Geometry check sheet. Reference: the model listing, model coordinates, mm. A direction names the side the tool comes from. Give positions to 0.01 mm unless a question says otherwise; leave off trailing zeros. Loops run counter-clockwise (first coordinate to the right, second up) from the corner with the lowest first, then second, coordinate; pieces in that order, holes last. Notation, with made-up numbers: (8.5, 37) -> (61.5, 37) arc R30 cw to (61.5, 61) -> close; hole circle Ø7 at (-6, 84.25). An arc over 180 degrees is marked (long way). Answer in a Markdown table with one row per item. Add a question column.
```python
from build123d import *

# Parameters (mm, degrees)
SKETCH1_R           = 5
BOSS_EXTRUDE1_DEPTH = 10
SKETCH2_R           = 8.5
BOSS_EXTRUDE2_DEPTH = 5
CUT_EXTRUDE1_DEPTH  = 3
CHAMFER1_SIZE       = 4


with BuildPart() as part:
    # Sketch1 → Boss-Extrude1 (new body)
    with BuildSketch(Plane.XY):
        Circle(SKETCH1_R)
    extrude(amount=BOSS_EXTRUDE1_DEPTH)

    # Sketch2 → Boss-Extrude2 (add)
    with BuildSketch(Plane.XY.offset(10)):
        Circle(SKETCH2_R)
    extrude(amount=BOSS_EXTRUDE2_DEPTH)

    # Sketch3 → Cut-Extrude1 (cut)
    with BuildSketch(Plane.XY.offset(15)):
        with BuildLine():
            Line((-2.8, 2.8), (2.8, 2.8))
            ThreePointArc((2.8, 2.8), (5.6, 0), (2.8, -2.8))
            Line((2.8, -2.8), (-2.8, -2.8))
            ThreePointArc((-2.8, -2.8), (-5.6, 0), (-2.8, 2.8))
        make_face()
    extrude(amount=-CUT_EXTRUDE1_DEPTH, mode=Mode.SUBTRACT)

    # Chamfer1
    # the kernel refuses this chamfer: 4 mm, written as the material it takes off along each edge
    with BuildSketch(Plane(origin=(0, 0, 10), x_dir=(1, 0, 0), z_dir=(0, -1, 0))) as chamfer1_piece_1_section:
        Polygon((8.5, CHAMFER1_SIZE), (8.5 - CHAMFER1_SIZE, 0), (8.5, 0), align=None)
    chamfer1_piece_1 = revolve(axis=Axis((0, 0, 10), (0, 0, 1)), mode=Mode.PRIVATE)
    chamfer1_piece_1 = chamfer1_piece_1 - Plane(origin=(0, 0, 12.254882924), x_dir=(1, 0, 0), z_dir=(0, 0, -1)) * Cylinder(5, 34, mode=Mode.PRIVATE)
    add(chamfer1_piece_1, mode=Mode.SUBTRACT)


solid = part.part
```
1. Access from +Z, -Z, +X, -X, +Y, -Y to the whole of each face (thin tool, end or side, straight path). Record for faces 1 (the face through (0, 0, 0)), 2 (the face through (0, 0, 12)).
2. Sectioned sample at A-A (y = 0). Enter the section's corners in (x, z).
3. Gauge pin test, flat ends, axial feed: pin 1 Ø3.5 at (x, z) = (0, 13.5) entering from -Y; pin 2 Ø6 at (y, z) = (-6.5, 6) entering from -X; pin 3 Ø6 at (x, y) = (-6.5, 6) entering from -Z; pin 4 Ø8 at (x, z) = (1, 5.5) entering from +Y. Record the tip position at first contact, or that the pin passes through.
4. Sectioned sample at C-C (z = 9). Enter the section's corners in (x, y).
5. Material ranges on L1, parallel to Y at x = 0.25, z = 12.5; L2, parallel to Y at x = -4.75, z = 12.75; L3, parallel to Z at x = -0.75, y = -2, recorded low to high. Write a range as from..to.
6. Release check for a two-part mould opening along Y. For faces 3 (the face through (4.57, 7.167, 14.493)), 4 (the face through (0, 2.8, 14)), 5 (the face through (0, -4, 15)) record: released by +Y, released by -Y, zero draft, split by the parting line, or undercut.
7. Sectioned sample at B-B (x = 0). Enter the section's corners in (y, z).
Response:
| question | item | result |
|---|---|---|
| 1 | face 1 | -Z, +X, -X, +Y, -Y |
| 1 | face 2 | +Z |
| 2 | outline | (-8.5, 14) -> (-5, 10.5) -> (-5, 0) -> (5, 0) -> (5, 10.5) -> (8.5, 14) -> (8.5, 15) -> (5.6, 15) -> (5.6, 12) -> (-5.6, 12) -> (-5.6, 15) -> (-8.5, 15) -> close |
| 3 | pin 1 | stops at y = -8.5 |
| 3 | pin 2 | stops at x = -3.57 |
| 3 | pin 3 | stops at z = 11.35 |
| 3 | pin 4 | stops at y = 5 |
| 4 | outline | circle Ø10 at (0, 0) |
| 5 | L1 | y = -7..-2.8, 2.8..7 |
| 5 | L2 | y = -5.48..-2.01, 2.01..5.48 |
| 5 | L3 | z = 0..12 |
| 6 | face 3 | split by the parting line |
| 6 | face 4 | undercut |
| 6 | face 5 | zero draft |
| 7 | outline | (-8.5, 14) -> (-5, 10.5) -> (-5, 0) -> (5, 0) -> (5, 10.5) -> (8.5, 14) -> (8.5, 15) -> (2.8, 15) -> (2.8, 12) -> (-2.8, 12) -> (-2.8, 15) -> (-8.5, 15) -> close |
